```python
from build123d import *

# Parameters (mm, degrees)
F0_W          = 2
F0_H          = 4
F0_H_2        = 2
F1_DEPTH      = 60
F1_DEPTH_BACK = 60


with BuildPart() as f1:
    # F0 (on Top) → F1 (new body, two sides)
    with BuildSketch(Plane.XY) as f1_sk:
        Polygon((-3, 30), (-5, 30), (-5, 23.5), (-5, -23.5), (-5, -30), (-3, -30), (0, -30), (0, 30), align=None)
        Polygon((-9, 30), (-5, 30), (-3, 30), (-3, 32), (-9, 32), align=None)
        with Locations((-10, 28)):
            Rectangle(F0_W, F0_H)
        with Locations((-10, 31)):
            Rectangle(F0_W, F0_H_2)
        Polygon((-3, -30), (-5, -30), (-9, -30), (-9, -32), (-3, -32), align=None)
        with Locations((-10, -31)):
            Rectangle(F0_W, F0_H_2)
        with Locations((-10, -28)):
            Rectangle(F0_W, F0_H)
    extrude(amount=F1_DEPTH)
    extrude(f1_sk.sketch, amount=-F1_DEPTH_BACK)


solid = f1.part
```
Here's how the part is built. I have some questions about the finished solid (model axes, mm). A direction names the side the tool comes from. Give positions to 0.01 mm unless a question says otherwise; leave off trailing zeros. Write each loop counter-clockwise with the first axis right and the second up, starting at its lowest first coordinate (ties: lowest second). Pieces come first, ordered by that corner, then holes. Notation, with made-up numbers: (47, 49) -> (72, 49) arc R33 cw to (72, 88) -> close; hole circle Ø4 at (35.25, 54). An arc over 180 degrees is marked (long way). Use one line per item in the form item = value.
1) On a 3-axis mill with a long thin cutter (end or side, diameter ignored), from which of +Z, -Z, +X, -X, +Y, -Y can I reach the whole of each face in a straight line? I mean faces 4 (the face through (-9, 28, 1)), 5 (the face through (-2, -30, 1)), 6 (the face through (0, 0, 1)). Say none if no direction works.
Verdict:
face_4 = +Z, -Z
face_5 = +Z, -Z, +X, -Y
face_6 = +Z, -Z, +X, +Y, -Y
2) If I drill on L1, parallel to X at y = 27.5, z = 20.5; L2, parallel to Y at x = -9.25, z = -21; L3, parallel to Y at x = -7.75, z = -17, over which ranges is the centre line in solid material (lowest first)? Write a range as [from, to].
Verdict:
L1 = [-11, -9], [-5, 0]
L2 = [-32, -26], [26, 32]
L3 = [-32, -30], [30, 32]
3) I'm going to push flat-ended pins straight in: pin 1 (1.5 mm diameter, centred on x = -7, y = 1.5, fed in from -Z); pin 2 (0.6 mm diameter, centred on y = -31.5, z = 9.5, fed in from +X); pin 3 (18 mm diameter, centred on y = -5.5, z = -28, fed in from -X). Where does each tip first touch, or does it pass through?
Verdict:
pin_1 = through
pin_2 = -3
pin_3 = -5
4) Suppose I cut it at C-C (y = 20). Please give me the cut outline in (x, z).
Verdict:
outline = (-5, -60) -> (0, -60) -> (0, 60) -> (-5, 60) -> close
5) Suppose I cut it at B-B (z = -10). Please give me the cut outline in (x, y), and give its area (3 significant figures).
Verdict:
outline = (-11, -32) -> (-3, -32) -> (-3, -30) -> (0, -30) -> (0, 30) -> (-3, 30) -> (-3, 32) -> (-11, 32) -> (-11, 26) -> (-9, 26) -> (-9, 30) -> (-5, 30) -> (-5, -30) -> (-9, -30) -> (-9, -26) -> (-11, -26) -> close
area = 348 mm2
6) We'd pull the mould along X, two halves only. Please class faces 1 (the face through (-1, 30, 1)), 2 (the face through (-7, 30, 1)), 3 (the face through (-11, -29, 1)): +X half, -X half, draft (parallel to the pull), parting line (faces both ways), or undercut.
Verdict:
face_1 = draft
face_2 = undercut
face_3 = -X half
7) Suppose I cut it at D-D (x = -1.25). Please give me the cut outline in (y, z).
Verdict:
outline = (-30, -60) -> (30, -60) -> (30, 60) -> (-30, 60) -> close
8) Suppose I cut it at A-A (x = -6.25). Please give me the cut outline in (y, z).
Verdict:
outline = (-32, -60) -> (-30, -60) -> (-30, 60) -> (-32, 60) -> close; (30, -60) -> (32, -60) -> (32, 60) -> (30, 60) -> close
